Here's how the part is built. I have some questions about the finished solid (model axes, mm). A direction names the side the tool comes from. Give positions to 0.01 mm unless a question says otherwise; leave off trailing zeros. Write each loop counter-clockwise with the first axis right and the second up, starting at its lowest first coordinate (ties: lowest second). Pieces come first, ordered by that corner, then holes. Notation, with made-up numbers: (7.25, 6.5) -> (17.25, 6.5) arc R30 ccw to (17.25, 36.5) -> close; hole circle Ø8 at (-10, 43). An arc over 180 degrees is marked (long way). Use one line per item in the form item = value.
```python
from build123d import *

# Parameters (mm, degrees)
SALIENTE_EXTRUIR1_DEPTH                              = 16
CROQUIS2_R                                           = 6.2
CORTAR_EXTRUIR1_DEPTH                                = 17
CROQUIS3_R                                           = 2
CORTAR_EXTRUIR2_DEPTH                                = 4
REFRENTADO_PARA_TORNILLO_TAP_N_CON_CABEZ_D           = 3.4
REFRENTADO_PARA_TORNILLO_TAP_N_CON_CABEZ_CSINK_D     = 6.72
REFRENTADO_PARA_TORNILLO_TAP_N_CON_CABEZ_CSINK_ANGLE = 90
CROQUIS6_R                                           = 3.5
CORTAR_EXTRUIR3_DEPTH                                = 10


with BuildPart() as part:
    # Croquis1 → Saliente-Extruir1 (new body)
    with BuildSketch(Plane.XY):
        Polygon((-121.785392746, 32.439983022), (-153.785392746, 32.439983022), (-166.785392746, 32.439983022), (-166.785392746, 6.439983022), (-121.785392746, 6.439983022), (-121.785392746, 10.439983022), (-146.785392746, 10.439983022), (-146.785392746, 29.439983022), (-121.785392746, 29.439983022), align=None)
    extrude(amount=SALIENTE_EXTRUIR1_DEPTH)

    # Croquis2 → Cortar-Extruir1 (cut)
    with BuildSketch(Plane.ZY.offset(166.785392746)):
        with Locations((8, 19.439983022)):
            Circle(CROQUIS2_R)
    extrude(amount=-CORTAR_EXTRUIR1_DEPTH, mode=Mode.SUBTRACT)

    # Croquis3 → Cortar-Extruir2 (cut)
    with BuildSketch(Plane.XZ.offset(-6.439983022)):
        with Locations((-131.785392746, 8)):
            Circle(CROQUIS3_R)
    extrude(amount=-CORTAR_EXTRUIR2_DEPTH, mode=Mode.SUBTRACT)

    # Refrentado para tornillo tapón con cabeza plana de clavija de M31 (through all)
    with Locations(Plane(origin=(0, 6.439983022, 0), x_dir=(-1, 0, 0), z_dir=(0, -1, 0))):
        with Locations((131.785392746, -8)):
            CounterSinkHole(REFRENTADO_PARA_TORNILLO_TAP_N_CON_CABEZ_D / 2, REFRENTADO_PARA_TORNILLO_TAP_N_CON_CABEZ_CSINK_D / 2, counter_sink_angle=REFRENTADO_PARA_TORNILLO_TAP_N_CON_CABEZ_CSINK_ANGLE)

    # Croquis6 → Cortar-Extruir3 (cut)
    with BuildSketch(Plane(origin=(0, 0, 0), x_dir=(-1, 0, 0), z_dir=(0, 0, -1))):
        with Locations((152.785392746, 19.439983022)):
            Circle(CROQUIS6_R)
    extrude(amount=-CORTAR_EXTRUIR3_DEPTH, mode=Mode.SUBTRACT)


solid = part.part
```
Q1. If I drill on line 1 along X through (y, z) = (30.7, 8); line 2 along Y through (x, z) = (-126.5, 9.5); line 3 along Y through (x, z) = (-156.25, 8), over which ranges is the centre line in solid material (lowest first)? Write a range as from..to.
Result set:
line_1 = -166.79..-133.49, -130.09..-121.79
line_2 = 6.44..10.44, 29.44..32.44
line_3 = 6.44..13.24, 25.64..32.44
Q2. Which directions (+Z, -Z, +X, -X, +Y, -Y) give clear straight access to the entire face, cutting with the end or side of a thin tool? Please do faces 1 (the face through (-133.783, 9.102, 8.088)), 2 (the face through (-158.4, 17.07, 13.73)), 3 (the face through (-146.785, 20, 8)).
Result set:
face_1 = -Y
face_2 = -X
face_3 = +Z, -Z, +X
Q3. I want a section at D-D, the plane z = 3. Write out the boundary of the cut face in (x, y), and give its area (3 significant figures).
Result set:
outline = (-166.79, 6.44) -> (-121.79, 6.44) -> (-121.79, 10.44) -> (-146.79, 10.44) -> (-146.79, 29.44) -> (-121.79, 29.44) -> (-121.79, 32.44) -> (-166.79, 32.44) -> (-166.79, 23.11) -> (-149.79, 23.11) -> (-149.79, 21.24) arc R3.5 cw to (-149.79, 17.64) -> (-149.79, 15.77) -> (-166.79, 15.77) -> close
area = 569 mm2
Q4. If we mould it in two halves opening along X, with no side actions, what happens to faces 4 (the face through (-149.286, 19.491, 3.495)), 5 (the face through (-149.785, 20, 11)), 6 (the face through (-155, 20, 16)), 7 (the face through (-130.164, 30.961, 7.489))? For each: +X half, -X half, draft (parallel to the pull), parting line (faces both ways), or undercut.
Result set:
face_4 = undercut
face_5 = -X half
face_6 = draft
face_7 = undercut
Q5. Will these pins go through, and if not, where does the flat tip stop? pin 1 Ø6.5 at (x, y) = (-152.79, 19.44) entering from -Z; pin 2 Ø5 at (y, z) = (18.5, 8.5) entering from -X; pin 3 Ø2.5 at (x, z) = (-131.79, 8) entering from +Y; pin 4 Ø5.5 at (x, z) = (-131.79, 8) entering from -Y.
Result set:
pin_1 = 10
pin_2 = -149.79
pin_3 = through
pin_4 = 7.05
Q6. I want a section at B-B, the plane z = 8. Write out the boundary of the cut face in (x, y).
Result set:
outline = (-166.79, 6.44) -> (-135.15, 6.44) -> (-133.79, 7.8) -> (-133.79, 10.44) -> (-146.79, 10.44) -> (-146.79, 29.44) -> (-133.49, 29.44) -> (-133.49, 32.44) -> (-166.79, 32.44) -> (-166.79, 25.64) -> (-149.79, 25.64) -> (-149.79, 21.24) arc R3.5 cw to (-149.79, 17.64) -> (-149.79, 13.24) -> (-166.79, 13.24) -> close; (-130.09, 29.44) -> (-121.79, 29.44) -> (-121.79, 32.44) -> (-130.09, 32.44) -> close; (-129.79, 7.8) -> (-128.43, 6.44) -> (-121.79, 6.44) -> (-121.79, 10.44) -> (-129.79, 10.44) -> close
Q7. I want a section at C-C, the plane y = 18.75. Write out the boundary of the cut face in (x, z), and give its area (3 significant figures).
Result set:
outline = (-166.79, 0) -> (-156.22, 0) -> (-156.22, 1.84) -> (-166.79, 1.84) -> close; (-166.79, 14.16) -> (-149.79, 14.16) -> (-149.79, 10) -> (-149.35, 10) -> (-149.35, 0) -> (-146.79, 0) -> (-146.79, 16) -> (-166.79, 16) -> close
area = 94.4 mm2
Q8. I want a section at A-A, the plane x = -141. Write out the boundary of the cut face in (y, z).
Result set:
outline = (6.44, 0) -> (10.44, 0) -> (10.44, 16) -> (6.44, 16) -> close; (29.44, 0) -> (32.44, 0) -> (32.44, 16) -> (29.44, 16) -> close
